from build123d import *

# Parameters (mm, degrees)
F0_W            = 160
F0_H            = 120
F1_DEPTH        = 25
F2_R            = 5
F4_DEPTH        = 40
F4_COPIES_COUNT = 9
F4_COPIES_ANGLE = 270


# Not quite as in the source:
# - a pattern or mirror of a feature is missing from the dataset's text; its kind, count and spacing are read off the source's solid


with BuildPart() as f1:
    # F0 (on Top) → F1 (new body)
    with BuildSketch(Plane.XY):
        with Locations((-35.207672789, -2.114020288)):
            Rectangle(F0_W, F0_H)
    extrude(amount=F1_DEPTH)

    # F2 (on face) → F4 (join)
    with BuildSketch(Plane.XY.offset(25)):
        with Locations((-75.6510049105, 21.4327722788)):
            Circle(F2_R)
    f4 = extrude(amount=F4_DEPTH)

    # F4_copies: F4 ×9 about axis
    f4_copies_axis = Axis((-35.207673, -2.11402, 0), (0, 0, -1))
    for i in range(1, F4_COPIES_COUNT):
        add(f4.rotate(f4_copies_axis, i * F4_COPIES_ANGLE / (F4_COPIES_COUNT - 1)))


solid = f1.part
Part model, mm, in its own coordinate system. A direction names the side the tool comes from. Give positions to 0.01 mm unless a question says otherwise; leave off trailing zeros. Order: outer loops, then holes, each group sorted by start corner. A loop starts at its lowest first (then second) coordinate and runs counter-clockwise, first axis right, second up. Notation, with made-up numbers: (42, -1.5) - (71, -1.5) arc R17 cw to (71, 11.5) - close; hole circle Ø9 at (-10.75, 19). An arc over 180 degrees is marked (long way). Use a Markdown table: item, result.
1) Two-plate mould, pull along Y, no slides. Class faces 1 (the cylindrical face through (4.15, -16.34, 44.72)), 2 (the flat face through (-36, 57.886, 12)), 3 (the flat face through (-115.208, -3, 12)): +Y half, -Y half, draft (parallel to the pull), parting line (faces both ways), or undercut.
Checked values:
| item | result |
|---|---|
| face 1 | undercut |
| face 2 | +Y half |
| face 3 | draft |
2) Saw through at C-C on x = -95.5. List the corners of the cut face in (y, z).
Checked values:
| item | result |
|---|---|
| outline | (-62.11, 0) - (57.89, 0) - (57.89, 25) - (-62.11, 25) - close |
3) Probe L1, parallel to Z at x = -77.5, y = -50.5; L2, parallel to X at y = 10, z = 52; L3, parallel to X at y = -45, z = 31. List the from-to ranges inside material, lowest first. Write a range as from..to.
Checked values:
| item | result |
|---|---|
| L1 | 0..25 |
| L2 | 5.04..15.04 |
| L3 | -63.12..-54.39, -35.54..-29.09 |
4) 3-axis set-ups, long thin cutter, end or side, ignore diameter. For faces 4 (the flat face through (44.792, -3, 12)), 5 (the cylindrical face through (7.355, 14.052, 44.72)): which of +Z, -Z, +X, -X, +Y, -Y reach the whole face in a straight line?
Checked values:
| item | result |
|---|---|
| face 4 | +Z, -Z, +X, +Y, -Y |
| face 5 | +Z |
5) Saw through at B-B on y = 42. List the corners of the cut face in (x, z), plus the area to 3 significant figures.
Checked values:
| item | result |
|---|---|
| outline | (-115.21, 0) - (44.79, 0) - (44.79, 25) - (-24.47, 25) - (-24.47, 65) - (-33.39, 65) - (-33.39, 25) - (-51.2, 25) - (-51.2, 65) - (-60.31, 65) - (-60.31, 25) - (-115.21, 25) - close |
| area | 4,720 mm² |
6) Flat gauge pins, fed straight in: P1, Ø2, axis at x = 11.5, y = 16, coming from the +Z side; P2, Ø1, axis at y = 8.5, z = 47.5, coming from the -X side; P3, Ø5, axis at y = -47, z = 45, coming from the +X side. Where does each tip first touch, or does it go through?
Checked values:
| item | result |
|---|---|
| P1 | z = 25 |
| P2 | x = 5.11 |
| P3 | x = -27.32 |
7) Saw through at A-A on z = 58. Count the separate pieces of the cut face and the enclosed holes in it, plus the area to 3 significant figures.
Checked values:
| item | result |
|---|---|
| separate pieces | 9 |
| enclosed holes | 0 |
| area | 707 mm² |
